from build123d import *

# Parameters (mm, degrees)
SKETCH_2_R               = 9.35
SKETCH_2_R_2             = 4.2
EXTRUDE_1_DEPTH          = 20
EXTRUDE_START            = -10
EXTRUDE_2_DEPTH          = 10
CUT_EXTRUDE_1_REACH      = 30.933
SKETCH_3_R               = 1.3
PATTERN_CIRCULAR_1_COUNT = 3
CUT_EXTRUDE_2_DEPTH      = 10
CHAMFER_1_SIZE           = 0.5


with BuildPart() as part:
    # Эскиз2 → Бобышка-Вытянуть1 (new body)
    with BuildSketch(Plane.XY):
        Circle(SKETCH_2_R)
        Circle(SKETCH_2_R_2, mode=Mode.SUBTRACT)
    extrude(amount=EXTRUDE_1_DEPTH)

    # Эскиз4 → Бобышка-Вытянуть2 (add)
    with BuildSketch(Plane.XY.offset(20).offset(EXTRUDE_START)):
        with BuildLine():
            Line((-2.833725463, 3.1), (2.833725463, 3.1))
            ThreePointArc((2.833725463, 3.1), (0, 4.2), (-2.833725463, 3.1))
        make_face()
    extrude(amount=EXTRUDE_2_DEPTH)

    # Эскиз3 → Вырез-Вытянуть1 (cut, up to next)
    with BuildSketch(Plane(origin=(0, 9.35, 0), x_dir=(1, 0, 0), z_dir=(0, 1, 0)), mode=Mode.PRIVATE) as cut_extrude_1_sk1:
        with Locations(Location((0, -16, 0), (0, 0, 270))):
            Circle(SKETCH_3_R)
    cut_extrude_1_tool1 = extrude(cut_extrude_1_sk1.sketch, amount=-CUT_EXTRUDE_1_REACH, mode=Mode.PRIVATE) & part.part
    cut_extrude_1 = cut_extrude_1_tool1.solids().sort_by_distance((0, 9.35, 16))[0]
    add(cut_extrude_1, mode=Mode.SUBTRACT)

    # Круговой массив1: Вырез-Вытянуть1 ×3 about axis
    pattern_circular_1_axis = Axis((0, 0, 20), (0, 0, -1))
    for i in range(1, PATTERN_CIRCULAR_1_COUNT):
        add(cut_extrude_1.rotate(pattern_circular_1_axis, i * 360 / PATTERN_CIRCULAR_1_COUNT), mode=Mode.SUBTRACT)

    # Эскиз5 → Вырез-Вытянуть2 (cut)
    with BuildSketch(Plane(origin=(0, 0, 0), x_dir=(-1, 0, 0), z_dir=(0, 0, -1))):
        with BuildLine():
            Line((-4.839679741, 8), (4.839679741, 8))
            ThreePointArc((4.839679741, 8), (0, 9.35), (-4.839679741, 8))
        make_face()
    extrude(amount=-CUT_EXTRUDE_2_DEPTH, mode=Mode.SUBTRACT)

    # Фаска1
    chamfer_1_edges = [part.edges().sort_by_distance(p)[0] for p in [
        (-4.591921951, -8.144737736, 0),
        (0, 8, 0),
    ]]
    chamfer(chamfer_1_edges, length=CHAMFER_1_SIZE)


solid = part.part
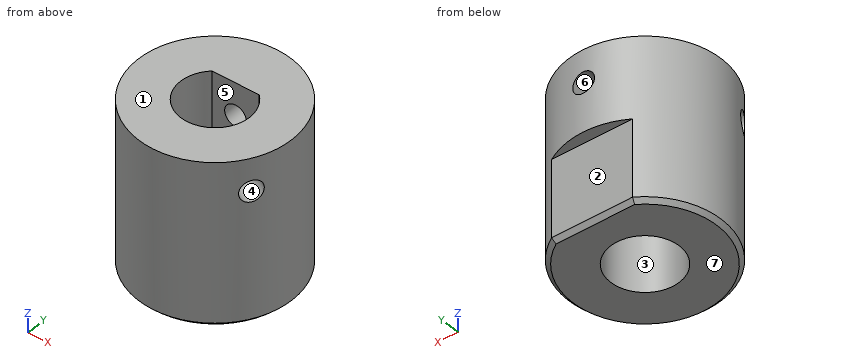
Build history of the part. All positions in model axes, mm. Face numbers are marked on the shaded views. A direction names the side the tool comes from. Round coordinates to 2 decimals unless told otherwise and drop trailing zeros. Loops run counter-clockwise (first coordinate to the right, second up) from the corner with the lowest first, then second, coordinate; pieces in that order, holes last. Notation, with made-up numbers: (22.5, -19.75) -> (31.5, -19.75) arc R26 ccw to (31.5, 7.25) -> close; hole circle Ø2 at (-11.5, 65). An arc over 180 degrees is marked (long way). Use CSV: the item, a comma, the result in double quotes. Start each with the question number.
Q1. Mould opens along Z. For the marked faces 4, 5, 6 and 7 say: +Z half, -Z half, draft (parallel to the pull), parting line (faces both ways), or undercut.
Q2. Saw through at C-C on z = 9.25. Give the cut face in (x, y), and give its area (3 significant figures).
Q3. Saw through at A-A on x = 0. Give the cut face in (y, z), and give its area (3 significant figures).
Q4. Saw through at B-B on z = 16. Give the cut face in (x, y), and give its area (3 significant figures).
Q5. Saw through at D-D on z = 18.5. Give the cut face in (x, y), and give its area (3 significant figures).
Q6. Flat gauge pins, fed straight in: pin 1 Ø5 at (x, z) = (-4.5, 2.5) entering from +Y; pin 2 Ø1.5 at (x, y) = (0.5, 8.5) entering from -Z; pin 3 Ø2 at (y, z) = (4, 6.5) entering from +X. Where does each tip first touch, or does it go through?
Q7. Which spindle directions (+Z, -Z, +X, -X, +Y, -Y) get a long thin tool onto all of the face, cutting with end or side? Do the marked faces 1, 2 and 3. Say none if no direction does.
Q8. Drill centre lines: L1, parallel to X at y = 0, z = 8; L2, parallel to Y at x = 0, z = 4; L3, parallel to Z at x = 0, y = 6.25. Where is each one in solid material? Low to high.
Solutions:
1,face 4,"undercut"
1,face 5,"draft"
1,face 6,"undercut"
1,face 7,"-Z half"
2,outline,"(-4.84, 8) arc R9.35 ccw (long way) to (4.84, 8) -> close; hole circle Ø8.4 at (0, 0)"
2,area,"210 mm^2"
3,outline,"(-9.35, 0.5) -> (-8.85, 0) -> (-4.2, 0) -> (-4.2, 20) -> (-9.35, 20) -> close; (3.1, 10) -> (4.2, 10) -> (4.2, 0) -> (7.5, 0) -> (8, 0.5) -> (8, 10) -> (9.35, 10) -> (9.35, 14.7) -> (3.1, 14.7) -> close; (3.1, 17.3) -> (9.35, 17.3) -> (9.35, 20) -> (3.1, 20) -> close"
3,area,"187 mm^2"
4,outline,"(-8.67, -3.5) -> (-4.11, -0.87) arc R4.2 cw to (-2.83, 3.1) -> (-1.3, 3.1) -> (-1.3, 9.26) arc R9.35 ccw to start; (-7.37, -5.76) arc R9.35 ccw to (7.37, -5.76) -> (2.81, -3.12) arc R4.2 cw to (-2.81, -3.12) -> close; (1.3, 3.1) -> (2.83, 3.1) arc R4.2 cw to (4.11, -0.87) -> (8.67, -3.5) arc R9.35 ccw to (1.3, 9.26) -> close"
4,area,"180 mm^2"
5,outline,"circle Ø18.7 at (0, 0); hole (-2.83, 3.1) arc R4.2 ccw (long way) to (2.83, 3.1) -> close"
5,area,"224 mm^2"
6,pin 1,"stops at y = 8"
6,pin 2,"stops at z = 0.25"
6,pin 3,"stops at x = 8.86"
7,face 1,"+Z, +X, -X, +Y, -Y"
7,face 2,"-Z, +X, -X, +Y"
7,face 3,"-Z"
8,L1,"x = -9.35 to -4.2, 4.2 to 9.35"
8,L2,"y = -9.35 to -4.2, 4.2 to 8"
8,L3,"z = 0 to 14.7, 17.3 to 20"
